Geometry check sheet. Reference: drawing and pictorial views, mm from the part's lowest x, y, z. A direction names the side the tool comes from. Coordinates: 2 decimals unless noted, no trailing zeros. Write each loop counter-clockwise with the first axis right and the second up, starting at its lowest first coordinate (ties: lowest second). Pieces come first, ordered by that corner, then holes. Notation, with made-up numbers: (-21.5, 89) -> (3.5, 89) arc R12 ccw to (3.5, 94) -> close; hole circle Ø1 at (-20.5, -4). An arc over 180 degrees is marked (long way). Put each result on its own line as item: value.
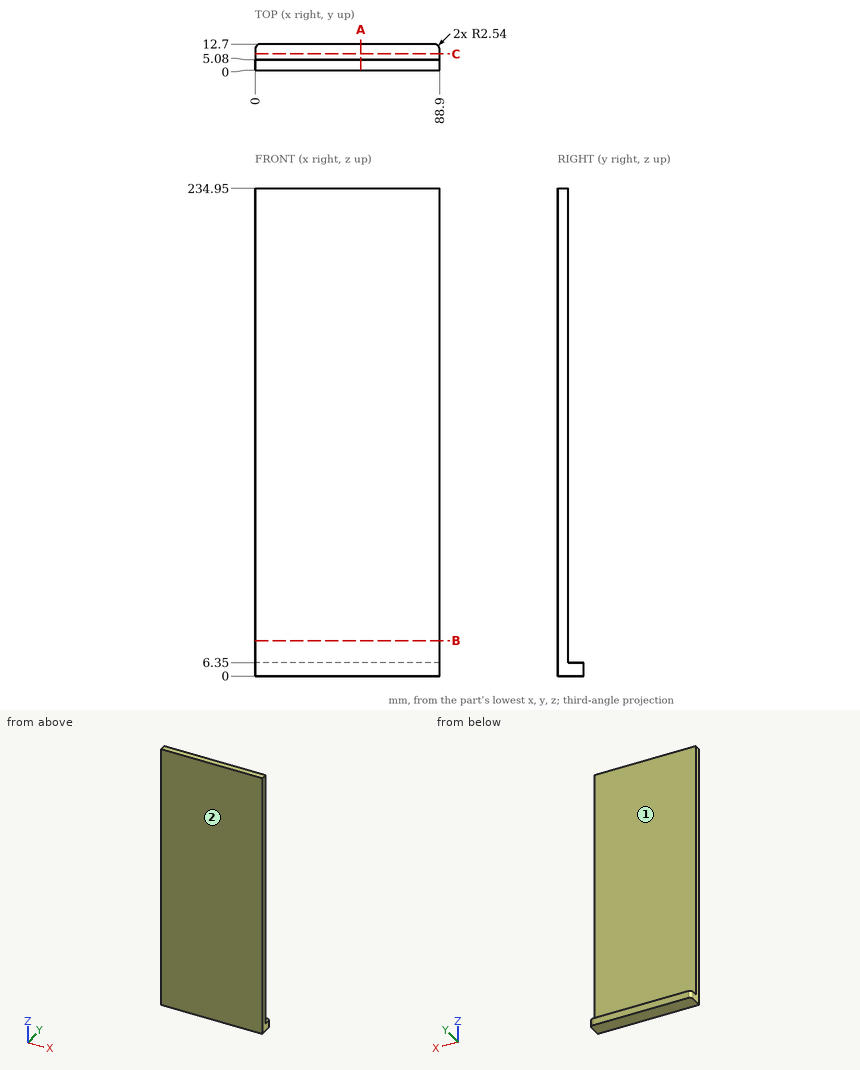
Q1. Tool access check on the marked faces 1 and 2. Record the directions out of +Z, -Z, +X, -X, +Y, -Y that give a thin tool (end or side, any length) a straight path to the whole face; none if there is none.
Recorded:
face 1: +Z, +X, -X, +Y
face 2: +Z, -Z, +X, -X, -Y
Q2. Cross-section at A-A (x = 51). Record the cut outline in (y, z), plus the area to 3 significant figures.
Recorded:
outline: (0, 0) -> (12.7, 0) -> (12.7, 6.35) -> (5.08, 6.35) -> (5.08, 234.95) -> (0, 234.95) -> close
area: 1,240 mm2
Q3. Cross-section at B-B (z = 17). Record the cut outline in (x, y), plus the area to 3 significant figures.
Recorded:
outline: (0, 0) -> (88.9, 0) -> (88.9, 5.08) -> (0, 5.08) -> close
area: 452 mm2
Q4. Material ranges on line 1 along Z through (x, y) = (7.5, 9); line 2 along Y through (x, z) = (36.5, 13.5), recorded low to high.
Recorded:
line 1: z = 0 to 6.35
line 2: y = 0 to 5.08
Q5. Depth check by flat-ended pin: P1, Ø8, axis at x = 36, z = 179, coming from the +Y side. Enter the tip coordinate at first touch or a pass-through.
Recorded:
P1: stops at y = 5.08
Q6. Cross-section at C-C (y = 8). Record the cut outline in (x, z).
Recorded:
outline: (0, 0) -> (88.9, 0) -> (88.9, 6.35) -> (0, 6.35) -> close
